Here's how the part is built. I have some questions about the finished solid (model axes, mm). Round coordinates to 2 decimals unless told otherwise and drop trailing zeros. Write each loop counter-clockwise with the first axis right and the second up, starting at its lowest first coordinate (ties: lowest second). Pieces come first, ordered by that corner, then holes. Notation, with made-up numbers: (6.25, 33) - (18.25, 33) arc R26 cw to (18.25, 54) - close; hole circle Ø7 at (72, -0.75). An arc over 180 degrees is marked (long way). Write item = value, one per line. Start each with the question number.
Item 1: If we section it at A-A (x = -34): Please give me the cut outline in (y, z).
Item 2: Thinking about a two-plate mould opening in X: for faces 1 (the face through (-1, -3, 0)), 2 (the face through (72, 0, 0)), 3 (the face through (-31.52, -0.54, 0.33)), 4 (the face through (-72, 0, 0)), which applies, pulls with the +X half, pulls with the -X half, needs draft (parallel to the pull), parting line crosses it, or undercut?
Item 3: If we section it at B-B (z = 0): Please give me the cut outline in (x, y).
Item 4: If I drill on line 1 along X through (y, z) = (-0.65, 0); line 2 along X through (y, z) = (-0.15, 2); line 3 along Z through (x, y) = (36, -1.25), over which ranges is the centre line in solid material (lowest first)? Write a range as [from, to].
```python
from build123d import *

# Parameters (mm, degrees)
SKETCH2_W                                         = 144
SKETCH2_H                                         = 20
BOSS_EXTRUDE1_DEPTH                               = 3
CSK_FOR_0_FLAT_HEAD_MACHINE_SCREW_100_D           = 4.999999906
CSK_FOR_0_FLAT_HEAD_MACHINE_SCREW_100_CSINK_D     = 6.99999997
CSK_FOR_0_FLAT_HEAD_MACHINE_SCREW_100_CSINK_ANGLE = 90


with BuildPart() as part:
    # Sketch2 → Boss-Extrude1 (new, symmetric)
    with BuildSketch(Plane(origin=(0, 0, 0), x_dir=(1, 0, 0), z_dir=(0, 1, 0))):
        Rectangle(SKETCH2_W, SKETCH2_H)
    extrude(amount=BOSS_EXTRUDE1_DEPTH, both=True)

    # CSK for #0 Flat Head Machine Screw (100)1 (through all)
    with Locations(Plane(origin=(-34, 3, 0), x_dir=(0, 0, 1), z_dir=(0, 1, 0))):
        with Locations((0, 0), (0, 70)):
            CounterSinkHole(CSK_FOR_0_FLAT_HEAD_MACHINE_SCREW_100_D / 2, CSK_FOR_0_FLAT_HEAD_MACHINE_SCREW_100_CSINK_D / 2, counter_sink_angle=CSK_FOR_0_FLAT_HEAD_MACHINE_SCREW_100_CSINK_ANGLE)


solid = part.part
```
Reply:
q1.outline = (-3, -10) - (3, -10) - (3, -3.5) - (2, -2.5) - (-3, -2.5) - close; (-3, 2.5) - (2, 2.5) - (3, 3.5) - (3, 10) - (-3, 10) - close
q2.face_1 = needs draft
q2.face_2 = pulls with the +X half
q2.face_3 = undercut
q2.face_4 = pulls with the -X half
q3.outline = (-72, -3) - (-36.5, -3) - (-36.5, 2) - (-37.5, 3) - (-72, 3) - close; (-31.5, -3) - (33.5, -3) - (33.5, 2) - (32.5, 3) - (-30.5, 3) - (-31.5, 2) - close; (38.5, -3) - (72, -3) - (72, 3) - (39.5, 3) - (38.5, 2) - close
q4.line_1 = [-72, -36.5], [-31.5, 33.5], [38.5, 72]
q4.line_2 = [-72, -35.5], [-32.5, 34.5], [37.5, 72]
q4.line_3 = [-10, -2.5], [2.5, 10]
